Part model, mm, in its own coordinate system. A direction names the side the tool comes from. Coordinates: 2 decimals unless noted, no trailing zeros. Loops run counter-clockwise (first coordinate to the right, second up) from the corner with the lowest first, then second, coordinate; pieces in that order, holes last.
```python
from build123d import *

# Parameters (mm, degrees)
F0_R        = 37.9287365184
F1_DEPTH    = 76.2
F3_R        = 20.4430640503
F4_DEPTH    = 43.688
F5_SIZE     = 2.54
F7_D        = 5.08
F8_T4_ANGLE = 68.0337710329
F8_S5_R     = 20.4430640503
F8_T6_DEPTH = 23


# Not quite as in the source:
# - a fillet or chamfer that OpenCascade refuses, or shapes differently, is made with other operations: its cross-section is extruded or revolved along the edge and cut away or added


with BuildPart() as f1:
    # F0 (on Front) → F1 (new body)
    with BuildSketch(Plane.XZ):
        Circle(F0_R)
    extrude(amount=F1_DEPTH)

    # F3 (on offset) → F4 (cut)
    with BuildSketch(Plane.XZ.offset(47.244)):
        with BuildLine():
            Line((-7.417100016, 52.0775169134), (-39.2948538065, 52.0775169134))
            Line((-39.2948538065, 52.0775169134), (-39.2948538065, 13.8873383403))
            Line((-39.2948538065, 13.8873383403), (-36.437637775, 13.8873383403))
            ThreePointArc((-36.437637775, 13.8873383403), (-15.9170187319, 22.3872570562), (-7.417100016, 42.9078760992))
            Line((-7.417100016, 42.9078760992), (-7.417100016, 52.0775169134))
        make_face()
        Polygon((43.7327071249, 2.8074141011), (57.5817332447, 26.8609896883), (43.6752387942, 50.8813859194), (15.9197182239, 50.8482065633), (2.070692104, 26.794630976), (15.9771865545, 2.7742347449), align=None)
        with Locations((-11.0355066136, -18.2179771364)):
            Circle(F3_R)
    extrude(amount=F4_DEPTH, mode=Mode.SUBTRACT)

    # F5
    f5_edges = [f1.edges().sort_by_distance(p)[0] for p in [
        (25.118202, -76.2, -28.419448),
        (37.902848, -76.2, 1.401132),
        (26.901202, -76.2, 2.787293),
        (9.023939, -76.2, 14.784433),
        (5.030877, -76.2, 31.936005),
        (-0.009512, -76.2, 37.928735),
        (-17.652727, -76.2, 20.787326),
        (-37.679979, -76.2, -4.336848),
        (-0.443827, -76.2, -0.732692),
    ]]
    chamfer(f5_edges, length=F5_SIZE)

    # F7 (through all)
    with Locations(Plane.XZ.offset(47.244)):
        with Locations((-11.6714835167, -7.6255151071), (0, -13.9276552945), (-14.5282614976, -18.8519991934), (-3.3601692412, -24.743270129), (-11.2020578235, -26.739705354), (-22.4352385849, -24.8684193939)):
            Hole(F7_D / 2)

    # F8: chamfer of 2.54 on 1 edges, made by hand


with BuildPart() as f8_tool2:
    # F8_s3 → F8_t4 (revolve)
    with BuildSketch(Plane(origin=(0, 0, 0), x_dir=(0, 1, 0), z_dir=(0.9987962472, 0, 0.0490515704))):
        Polygon((-44.704, -37.9287365184), (-47.244, -35.3887365184), (-47.244, -37.9287365184), align=None)
    revolve(axis=Axis((0, -47.244, 0), (0, 1, 0)), revolution_arc=F8_T4_ANGLE)

    # F8_s5 → F8_t6 (intersect, symmetric)
    with BuildSketch(Plane.XZ.offset(46)):
        with Locations((-11.0355066136, -18.2179771364)):
            Circle(F8_S5_R)
    extrude(amount=F8_T6_DEPTH, both=True, mode=Mode.INTERSECT)


with BuildPart() as f1_1:
    add(f1.part)

    # F8_t1: cut F8_tool2
    add(f8_tool2.part, mode=Mode.SUBTRACT)


solid = f1_1.part
```
Q1. Drop flat-ended pins along their axis: P1, Ø5, axis at y = -14, z = 25, coming from the -X side; P2, Ø11.5, axis at x = -19.5, z = 28.5, coming from the -Y side; P3, Ø1.5, axis at x = 21.5, y = -38.5, coming from the -Z side; P4, Ø2, axis at x = 3.5, z = 1, coming from the +Y side. Give the stop position or say it passes through.
Q2. Tool access for faces 1 (the conical face through (-36.08, -75.51, 0.04)), 2 (the cylindrical face through (0.11, -58.98, -1.08)), 3 (the flat face through (8.017, -74.948, 13.953)): list every direction of +Z, -Z, +X, -X, +Y, -Y with a clear straight run to the whole face (end or side of a thin tool).
Q3. Saw through at A-A (y = -64). List the corners of the cut face in (x, z).
Q4. Mould opens along Z. For faces 4 (the flat face through (-22, -47.244, 26)), 5 (the cylindrical face through (-17.859, -60.267, 20.614)), 6 (the flat face through (-11, -47.244, -16)) say: released by +Z, released by -Z, zero draft, split by the parting line, or undercut.
Q5. Probe line 1 (Z direction, x = 0, y = -20); line 2 (X direction, y = -31, z = -25); line 3 (Z direction, x = -10.5, y = -23). List the from-to ranges inside material, lowest first.
Q6. Saw through at B-B (y = -6). List the corners of the cut face in (x, z), plus the area to 3 significant figures.
Checked values:
1. P1: stops at x = -30.53
1. P2: stops at y = -47.24
1. P3: stops at z = -31.75
1. P4: stops at y = 0
2. face 1: -X, -Y
2. face 2: -Y
2. face 3: +X, -Y
3. outline: (-35.29, 13.91) arc R37.93 ccw to (-31.2, -21.56) arc R20.44 cw (long way) to (-4.66, -37.64) arc R37.93 ccw to (37.83, 2.8) - (15.98, 2.77) - (2.07, 26.79) - (7.99, 37.08) arc R37.93 ccw to (-8.01, 37.07) arc R29.02 cw to start
4. face 4: zero draft
4. face 5: released by +Z
4. face 6: undercut
5. line 1: z = -37.93 to -16.47, -11.39 to 37.93
5. line 2: x = -28.52 to -24.97, -19.9 to -13.05, -9.35 to -5.89, -0.83 to 28.52
5. line 3: z = -36.45 to -29.18, -24.3 to -9.88, -5.37 to 36.45
6. outline: circle Ø75.86 at (0, 0); hole circle Ø5.08 at (-22.44, -24.87); hole circle Ø5.08 at (-14.53, -18.85); hole circle Ø5.08 at (-11.67, -7.63); hole circle Ø5.08 at (-11.2, -26.74); hole circle Ø5.08 at (-3.36, -24.74); hole circle Ø5.08 at (0, -13.93)
6. area: 4,400 mm2
